from build123d import *

# Parameters (mm, degrees)
SKETCH1_W           = 45
SKETCH1_H           = 23.6
SKETCH1_R           = 1.75
BOSS_EXTRUDE1_DEPTH = 10
SKETCH2_R           = 1
SKETCH2_W           = 4
SKETCH2_H           = 8
CUT_EXTRUDE1_DEPTH  = 46
FILLET1_R           = 0.25
CHAMFER1_SIZE       = 0.2
SKETCH3_W           = 11.00513931
SKETCH3_H           = 32.516866569
SKETCH3_W_2         = 10
SKETCH3_H_2         = 36.117344973
CUT_EXTRUDE2_DEPTH  = 10


with BuildPart() as part:
    # Sketch1 → Boss-Extrude1 (new body)
    with BuildSketch(Plane.XY):
        Rectangle(SKETCH1_W, SKETCH1_H)
        with Locations((-12.5, 7.5)):
            Circle(SKETCH1_R, mode=Mode.SUBTRACT)
        with Locations((12.5, 7.5)):
            Circle(SKETCH1_R, mode=Mode.SUBTRACT)
        with Locations((12.5, -7.5)):
            Circle(SKETCH1_R, mode=Mode.SUBTRACT)
        with Locations((-12.5, -7.5)):
            Circle(SKETCH1_R, mode=Mode.SUBTRACT)
    extrude(amount=BOSS_EXTRUDE1_DEPTH)

    # Sketch2 → Cut-Extrude1 (cut, through all)
    with BuildSketch(Plane(origin=(22.5, 0, 0), x_dir=(0, 0, -1), z_dir=(1, 0, 0))):
        with Locations((-8, 4)):
            Circle(SKETCH2_R)
        with Locations((-8, -4)):
            Circle(SKETCH2_R)
        with Locations((-8, 0)):
            Rectangle(SKETCH2_W, SKETCH2_H)
    extrude(amount=-CUT_EXTRUDE1_DEPTH, mode=Mode.SUBTRACT)

    # Fillet1
    fillet1_edges = [part.edges().sort_by_distance(p)[0] for p in [
        (22.5, -7.9, 10),
        (0, 11.8, 10),
        (22.5, 7.9, 10),
        (-22.5, -7.9, 10),
        (0, -4, 10),
        (-22.5, 7.9, 10),
        (0, 4, 10),
        (0, 11.8, 0),
        (22.5, 0, 0),
        (0, -11.8, 0),
        (-22.5, 0, 0),
        (0, -11.8, 10),
        (-22.5, 11.8, 5),
        (22.5, 11.8, 5),
        (22.5, -11.8, 5),
        (-22.5, -11.8, 5),
    ]]
    fillet(fillet1_edges, radius=FILLET1_R)

    # Chamfer1
    chamfer1_edges = [part.edges().sort_by_distance(p)[0] for p in [
        (-14.25, 7.5, 0),
        (-14.25, 7.5, 10),
        (10.75, 7.5, 0),
        (10.75, 7.5, 10),
        (10.75, -7.5, 0),
        (10.75, -7.5, 10),
        (-14.25, -7.5, 0),
        (-14.25, -7.5, 10),
    ]]
    chamfer(chamfer1_edges, length=CHAMFER1_SIZE)

    # Sketch3 → Cut-Extrude2 (cut)
    with BuildSketch(Plane(origin=(0, 0, 0), x_dir=(-1, 0, 0), z_dir=(0, 0, -1))):
        with Locations((-20.552569655, 1.232790519)):
            Rectangle(SKETCH3_W, SKETCH3_H)
        with Locations((20.05, -0.567448683)):
            Rectangle(SKETCH3_W_2, SKETCH3_H_2)
    extrude(amount=-CUT_EXTRUDE2_DEPTH, mode=Mode.SUBTRACT)


solid = part.part
Work out the finished part from the listing and answer in its coordinate system (mm). A direction names the side the tool comes from. Give positions to 0.01 mm unless a question says otherwise; leave off trailing zeros. Order: outer loops, then holes, each group sorted by start corner. A loop starts at its lowest first (then second) coordinate and runs counter-clockwise, first axis right, second up. Notation, with made-up numbers: M -30,-12.75 L 24,-12.75 A12 ccw 24,3.25 Z; hole C -23.75,-5.75 d9. An arc over 180 degrees is marked long. Return JSON: item names as keys, results as strings.
Q1. The mould has two halves that part along Z. Classify faces 3 (the face through (15.05, 0, 5)), 4 (the face through (0, -5, 8)), 5 (the face through (0, 8, 10)): pulls with the +Z half, pulls with the -Z half, needs draft (parallel to the pull), parting line crosses it, or undercut.
Answer below:
{"face 3": "needs draft", "face 4": "undercut", "face 5": "pulls with the +Z half"}
Q2. Which of the six approach directions +Z, -Z, +X, -X, +Y, -Y give full straight-line access (tool end or side, diameter ignored) to faces 1 (the face through (0, 0, 0)), 2 (the face through (0.2, 4, 6.5))?
Answer below:
{"face 1": "-Z, +X, -X, +Y, -Y", "face 2": "+Z, +X, -X"}
Q3. Find section A-A, the plane y = -7.5. Write down the section's boundary in (x, z).
Answer below:
{"outline": "M -15.05,0 L -14.45,0 L -14.25,0.2 L -14.25,9.8 L -14.45,10 L -15.05,10 Z; M -10.75,0.2 L -10.55,0 L 10.55,0 L 10.75,0.2 L 10.75,9.8 L 10.55,10 L -10.55,10 L -10.75,9.8 Z; M 14.25,0.2 L 14.45,0 L 15.05,0 L 15.05,10 L 14.45,10 L 14.25,9.8 Z"}
Q4. Find section B-B, the plane z = 2.5. Write down the section's boundary in (x, y), and give its area (3 significant figures).
Answer below:
{"outline": "M -15.05,-11.8 L 15.05,-11.8 L 15.05,11.8 L -15.05,11.8 Z; hole C -12.5,-7.5 d3.5; hole C -12.5,7.5 d3.5; hole C 12.5,-7.5 d3.5; hole C 12.5,7.5 d3.5", "area": "672 mm^2"}
Q5. Find section C-C, the plane x = -12.5. State how many separate pieces and enclosed holes the cut face has, and give its area (3 significant figures).
Answer below:
{"separate pieces": "3", "enclosed holes": "0", "area": "131 mm^2"}
Q6. Each of these flat-tipped pins is pushed along its axis until it touches: pin 1 (3 mm diameter, centred on x = 12.5, y = 7.5, fed in from +Z); pin 2 (5 mm diameter, centred on y = 0.5, z = 6.5, fed in from -X); pin 3 (5 mm diameter, centred on x = -6, y = -0.5, fed in from +Z). Where does it stop, or does it pass through?
Answer below:
{"pin 1": "passes through", "pin 2": "stops at x = -15.05", "pin 3": "stops at z = 6"}
Q7. Find section D-D, the plane x = -2. Write down the section's boundary in (y, z).
Answer below:
{"outline": "M -11.8,0.25 A0.25 ccw -11.55,0 L 11.55,0 A0.25 ccw 11.8,0.25 L 11.8,9.75 A0.25 ccw 11.55,10 L 4.25,10 A0.25 ccw 4,9.75 L 4,9 A1 cw 4,7 L 4,6 L -4,6 L -4,7 A1 cw -4,9 L -4,9.75 A0.25 ccw -4.25,10 L -11.55,10 A0.25 ccw -11.8,9.75 Z"}
Q8. Find the intervals of material crossed by line 1 along Y through (x, z) = (-12.5, 6.5); line 2 along Y through (x, z) = (12.5, 4.75); line 3 along Y through (x, z) = (12.5, 8.75), in increasing order. Write a range as [from, to].
Answer below:
{"line 1": "y = [-11.8, -9.25], [-5.75, -4], [4, 5.75], [9.25, 11.8]", "line 2": "y = [-11.8, -9.25], [-5.75, 5.75], [9.25, 11.8]", "line 3": "y = [-11.8, -9.25], [-5.75, -4.66], [4.66, 5.75], [9.25, 11.8]"}
